Work out the finished part from the listing and answer in its coordinate system (mm). A direction names the side the tool comes from. Coordinates: 2 decimals unless noted, no trailing zeros. Loops run counter-clockwise (first coordinate to the right, second up) from the corner with the lowest first, then second, coordinate; pieces in that order, holes last. Notation, with made-up numbers: (-34, 26.5) -> (-8, 26.5) arc R23 cw to (-8, 62.5) -> close; hole circle Ø11 at (65, 1.5). An arc over 180 degrees is marked (long way). Use a Markdown table: item, result.
from build123d import *

# Parameters (mm, degrees)
F0_W     = 600
F0_H     = 540
F1_DEPTH = 18
F0_H_2   = 2000
F2_DEPTH = 18
F4_DEPTH = 2540


with BuildPart() as f1:
    # F0 (on Right) → F1 (new body)
    with BuildSketch(Plane.YZ):
        with Locations((0, 1000)):
            Rectangle(F0_W, F0_H)
    extrude(amount=F1_DEPTH)

    # F0 (on Right) → F2 (join)
    with BuildSketch(Plane.YZ):
        with Locations((0, -270)):
            Rectangle(F0_W, F0_H_2)
    extrude(amount=F2_DEPTH)

    # F3 (on face) → F4 (join)
    with BuildSketch(Plane.XY.offset(1270)):
        Polygon((18, -300), (0, -300), (-10, -310), (-10, -315), (28, -315), (28, -310), align=None)
    extrude(amount=-F4_DEPTH)


solid = f1.part
Q1. For faces 1 (the flat face through (0, -4, 18)), 2 (the flat face through (18, -4, 18)), determine the directions among +Z, -Z, +X, -X, +Y, -Y from which every point of the face is accessible in a straight line to the end or side of a thin tool.
Solved:
| item | result |
|---|---|
| face 1 | +Z, -Z, -X, +Y |
| face 2 | +Z, -Z, +X, +Y |
Q2. Section B-B on y = -266.5 is taken. Determine the outline of the cut face in (x, z), and give its area (3 significant figures).
Solved:
| item | result |
|---|---|
| outline | (0, -1270) -> (18, -1270) -> (18, 1270) -> (0, 1270) -> close |
| area | 45,700 mm² |
Q3. Section A-A on z = -985 is taken. Determine the outline of the cut face in (x, y).
Solved:
| item | result |
|---|---|
| outline | (-10, -315) -> (28, -315) -> (28, -310) -> (18, -300) -> (18, 300) -> (0, 300) -> (0, -300) -> (-10, -310) -> close |
Q4. Consider line 1 (X direction, y = 98, z = -436); line 2 (Y direction, x = 20, z = 850.5). Determine where each line is inside the solid, lowest interval first. Write a range as [from, to].
Solved:
| item | result |
|---|---|
| line 1 | [0, 18] |
| line 2 | [-315, -302] |
Q5. Given pin 1 Ø4 at (y, z) = (-176.5, -720) entering from -X; pin 2 Ø12 at (y, z) = (-112, -887) entering from +X, each flat-ended and moving along its own axis, determine where each tip first touches the part or whether it passes through.
Solved:
| item | result |
|---|---|
| pin 1 | x = 0 |
| pin 2 | x = 18 |
